```python
from build123d import *

# Parameters (mm, degrees)
SKETCH1_R           = 13.5
SKETCH1_R_2         = 3.75
BOSS_EXTRUDE1_DEPTH = 2.5
CUT_EXTRUDE1_DEPTH  = 20.254869514
CIRPATTERN1_COUNT   = 5
CHAMFER1_SIZE       = 0.5
SKETCH4_R           = 13.5
SKETCH4_R_2         = 13
CUT_EXTRUDE3_DEPTH  = 1.5


with BuildPart() as part:
    # Sketch1 → Boss-Extrude1 (new, symmetric)
    with BuildSketch(Plane(origin=(0, 0, 0), x_dir=(0, 0, -1), z_dir=(1, 0, 0))):
        Circle(SKETCH1_R)
        Circle(SKETCH1_R_2, mode=Mode.SUBTRACT)
    extrude(amount=BOSS_EXTRUDE1_DEPTH, both=True)

    # Sketch2 → Cut-Extrude1 (cut, symmetric)
    with BuildSketch(Plane(origin=(0, 0, 0), x_dir=(0, 0, -1), z_dir=(1, 0, 0))):
        with BuildLine():
            ThreePointArc((0, 5.849695328), (-2.956289657, 7.377375059), (-5.012219469, 9.99397715))
            ThreePointArc((-5.012219469, 9.99397715), (-2.621563936, 11.159720287), (0, 11.6087119))
            ThreePointArc((0, 11.6087119), (2.621563936, 11.159720287), (5.012219469, 9.99397715))
            ThreePointArc((5.012219469, 9.99397715), (2.956289657, 7.377375059), (0, 5.849695328))
        make_face()
    cut_extrude1 = extrude(amount=CUT_EXTRUDE1_DEPTH, both=True, mode=Mode.SUBTRACT)

    # CirPattern1: Cut-Extrude1 ×5 about axis
    cirpattern1_axis = Axis((0, 0, 0), (1, 0, 0))
    for i in range(1, CIRPATTERN1_COUNT):
        add(cut_extrude1.rotate(cirpattern1_axis, i * 360 / CIRPATTERN1_COUNT), mode=Mode.SUBTRACT)

    # Chamfer1
    chamfer1_edges = [part.edges().sort_by_distance(p)[0] for p in [
        (2.5, 0, 13.5),
        (2.5, 0, 3.75),
    ]]
    chamfer(chamfer1_edges, length=CHAMFER1_SIZE)

    # Sketch4 → Cut-Extrude3 (cut, symmetric)
    with BuildSketch(Plane(origin=(0, 0, 0), x_dir=(0, 0, -1), z_dir=(1, 0, 0))):
        Circle(SKETCH4_R)
        Circle(SKETCH4_R_2, mode=Mode.SUBTRACT)
    extrude(amount=CUT_EXTRUDE3_DEPTH, both=True, mode=Mode.SUBTRACT)


solid = part.part
```
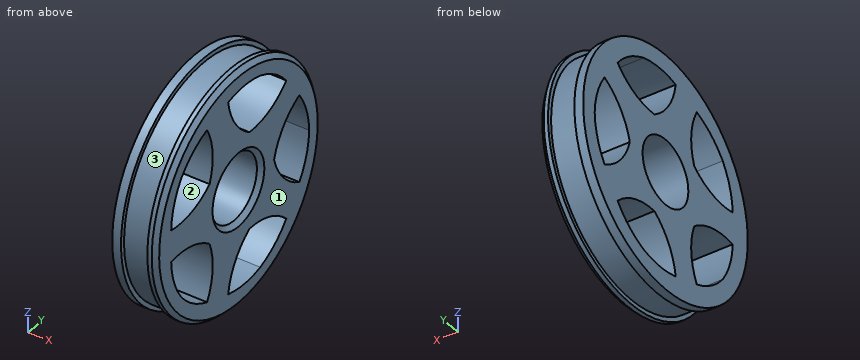
Geometry check sheet. Reference: the model listing, model coordinates, mm. Face numbers are marked on the shaded views. Give positions to 0.01 mm unless a question says otherwise; leave off trailing zeros. Order: outer loops, then holes, each group sorted by start corner. A loop starts at its lowest first (then second) coordinate and runs counter-clockwise, first axis right, second up.
1. Section check A-A, the plane x = 0.6. Enter the section's corners in (y, z), and give its area (3 significant figures).
2. Thickness scan on L1, parallel to Z at x = -0.4, y = -9.75; L2, parallel to Y at x = -1.85, z = -1; L3, parallel to Y at x = 0.1, z = -3.25. Record the ranges inside material, lowest first.
3. Section check B-B, the plane y = 0. Enter the section's corners in (x, z), and give its area (3 significant figures).
4. Gauge pin test, flat end, axial feed: pin 1 Ø1.5 at (x, y) = (0.5, -7.5) entering from +Z. Record the tip position at first contact, or that the pin passes through.
5. Section check C-C, the plane z = 6.25. Give the number of separate pieces and of enclosed holes in the cut face, and give its area (3 significant figures).
6. Release check for a two-part mould opening along Z. For the marked faces 1, 2 and 3 record: pulls with the +Z half, pulls with the -Z half, needs draft (parallel to the pull), parting line crosses it, or undercut.
Values follow:
1. outline: circle Ø26 at (0, 0); hole (-11.03, -1.82) arc R9.39 ccw to (-9.39, -6.82) arc R9.39 ccw to (-5.14, -9.93) arc R7.84 ccw to (-4.73, -3.44) arc R7.84 ccw to start; hole (-11.03, 1.82) arc R7.84 ccw to (-4.73, 3.44) arc R7.84 ccw to (-5.14, 9.93) arc R9.39 ccw to (-9.39, 6.82) arc R9.39 ccw to start; hole circle Ø7.5 at (0, 0); hole (-1.68, -11.05) arc R9.39 ccw to (3.59, -11.04) arc R9.39 ccw to (7.86, -7.96) arc R7.84 ccw to (1.81, -5.56) arc R7.84 ccw to start; hole (-1.68, 11.05) arc R7.84 ccw to (1.81, 5.56) arc R7.84 ccw to (7.86, 7.96) arc R9.39 ccw to (3.59, 11.04) arc R9.39 ccw to start; hole (5.85, 0) arc R7.84 ccw to (9.99, -5.01) arc R9.39 ccw to (11.61, 0) arc R9.39 ccw to (9.99, 5.01) arc R7.84 ccw to start
1. area: 298 mm2
2. L1: z = -8.6 to -6.26, -1.7 to 1.7, 6.26 to 8.6
2. L2: y = -13.46 to -3.61, 3.61 to 6.19, 11.53 to 13.46
2. L3: y = -12.59 to -10.87, -4.98 to -1.87, 1.87 to 7.63, 10.93 to 12.59
3. outline: (-2.5, -13.5) - (-1.5, -13.5) - (-1.5, -13) - (1.5, -13) - (1.5, -13.5) - (2, -13.5) - (2.5, -13) - (2.5, -11.38) - (-2.5, -11.38) - close; (-2.5, -7.19) - (2.5, -7.19) - (2.5, -4.25) - (2, -3.75) - (-2.5, -3.75) - close; (-2.5, 3.75) - (2, 3.75) - (2.5, 4.25) - (2.5, 7.19) - (-2.5, 7.19) - close; (-2.5, 11.38) - (2.5, 11.38) - (2.5, 13) - (2, 13.5) - (1.5, 13.5) - (1.5, 13) - (-1.5, 13) - (-1.5, 13.5) - (-2.5, 13.5) - close
3. area: 52.1 mm2
4. pin 1: stops at z = 11.11
5. separate pieces: 3
5. enclosed holes: 0
5. area: 65.6 mm2
6. face 1: needs draft
6. face 2: undercut
6. face 3: parting line crosses it
